from build123d import *

# Parameters (mm, degrees)
SKETCH1_W                   = 50.8
SKETCH1_H                   = 25.4
BOSS_EXTRUDE1_DEPTH         = 266.7
SKETCH2_W                   = 44.45
SKETCH2_H                   = 19.05
CUT_EXTRUDE1_DEPTH          = 535.155417458
SKETCH5_R                   = 2.4892
SKETCH5_R_2                 = 9.84885
SKETCH5_R_3                 = 14.2875
CUT_EXTRUDE2_DEPTH          = 508
SKETCH7_R                   = 6.35
CUT_EXTRUDE4_DEPTH          = 270.108175275
F_27_0_144_DIAMETER_HOLE1_D = 3.6576


with BuildPart() as part:
    # Sketch1 → Boss-Extrude1 (new, symmetric)
    with BuildSketch(Plane.XY):
        Rectangle(SKETCH1_W, SKETCH1_H)
    extrude(amount=BOSS_EXTRUDE1_DEPTH, both=True)

    # Sketch2 → Cut-Extrude1 (cut, through all)
    with BuildSketch(Plane.XY.offset(266.7)):
        Rectangle(SKETCH2_W, SKETCH2_H)
    extrude(amount=-CUT_EXTRUDE1_DEPTH, mode=Mode.SUBTRACT)

    # Sketch5 → Cut-Extrude2 (cut)
    with BuildSketch(Plane(origin=(0, 12.7, 0), x_dir=(1, 0, 0), z_dir=(0, 1, 0))):
        with Locations(Location((0, -260.35, 0), (0, 0, 270))):
            Circle(SKETCH5_R)
        with Locations(Location((0, -234.95, 0), (0, 0, 270))):
            Circle(SKETCH5_R_2)
        with Locations(Location((0, -209.55, 0), (0, 0, 270))):
            Circle(SKETCH5_R)
        with Locations(Location((0, 241.3, 0), (0, 0, 270))):
            Circle(SKETCH5_R_3)
    extrude(amount=-CUT_EXTRUDE2_DEPTH, mode=Mode.SUBTRACT)

    # Sketch7 → Cut-Extrude4 (cut, through all)
    with BuildSketch(Plane(origin=(0, 12.7, 0), x_dir=(1, 0, 0), z_dir=(0, 1, 0))):
        with Locations(Location((0, -107.95, 0), (0, 0, 270))):
            Circle(SKETCH7_R)
    extrude(amount=-CUT_EXTRUDE4_DEPTH, mode=Mode.SUBTRACT)

    # #27 (0.144) Diameter Hole1 (through all)
    with Locations(Plane(origin=(25.4, 0, 0), x_dir=(0, 0, -1), z_dir=(1, 0, 0))):
        with Locations((-247.65, 0), (-228.6, 0)):
            Hole(F_27_0_144_DIAMETER_HOLE1_D / 2)


solid = part.part
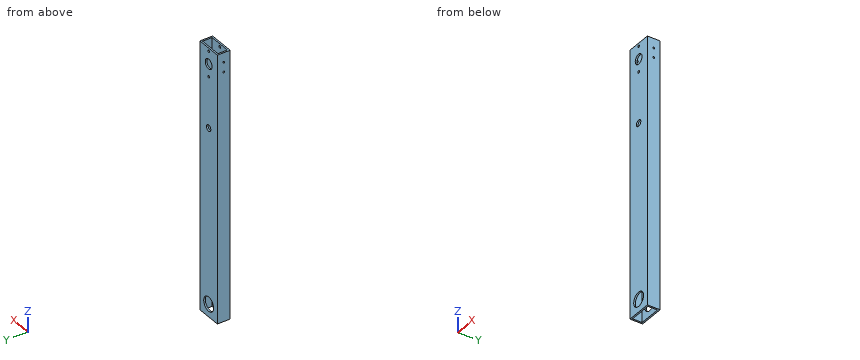
Work out the finished part from the listing and answer in its coordinate system (mm). Round coordinates to 2 decimals unless told otherwise and drop trailing zeros. Write each loop counter-clockwise with the first axis right and the second up, starting at its lowest first coordinate (ties: lowest second). Pieces come first, ordered by that corner, then holes. Notation, with made-up numbers: M 58,88 L 69,88 A18 ccw 69,115 Z; hole C 81,-38 d5. An arc over 180 degrees is marked long. Use a Markdown table: item, result.
1) Consider line 1 (X direction, y = 8, z = -156.5) (3 decimals); line 2 (Y direction, x = 4, z = -218.5) (3 decimals); line 3 (Y direction, x = -23.4, z = 228.6). Determine where each line is inside the solid, lowest interval first. Write a range as [from, to].
Taken from the geometry:
| item | result |
|---|---|
| line 1 | x = [-25.4, -22.225], [22.225, 25.4] |
| line 2 | y = [-12.7, -9.525], [9.525, 12.7] |
| line 3 | y = [-12.7, -1.83], [1.83, 12.7] |
2) The part is cut by section A-A on z = 234.95. Give the vertices of the cut face in (x, y) (3 decimals).
Taken from the geometry:
| item | result |
|---|---|
| outline | M -25.4,-12.7 L -9.849,-12.7 L -9.849,-9.525 L -22.225,-9.525 L -22.225,9.525 L -9.849,9.525 L -9.849,12.7 L -25.4,12.7 Z; M 9.849,-12.7 L 25.4,-12.7 L 25.4,12.7 L 9.849,12.7 L 9.849,9.525 L 22.225,9.525 L 22.225,-9.525 L 9.849,-9.525 Z |
3) The part is cut by section B-B on z = -166. Give the vertices of the cut face in (x, y) (3 decimals), plus the area to 3 significant figures.
Taken from the geometry:
| item | result |
|---|---|
| outline | M -25.4,-12.7 L 25.4,-12.7 L 25.4,12.7 L -25.4,12.7 Z; hole M -22.225,-9.525 L 22.225,-9.525 L 22.225,9.525 L -22.225,9.525 Z |
| area | 444 mm2 |
4) The part is cut by section C-C on z = -241.3. Give the vertices of the cut face in (x, y) (1 decimal).
Taken from the geometry:
| item | result |
|---|---|
| outline | M -25.4,-12.7 L -14.3,-12.7 L -14.3,-9.5 L -22.2,-9.5 L -22.2,9.5 L -14.3,9.5 L -14.3,12.7 L -25.4,12.7 Z; M 14.3,-12.7 L 25.4,-12.7 L 25.4,12.7 L 14.3,12.7 L 14.3,9.5 L 22.2,9.5 L 22.2,-9.5 L 14.3,-9.5 Z |
